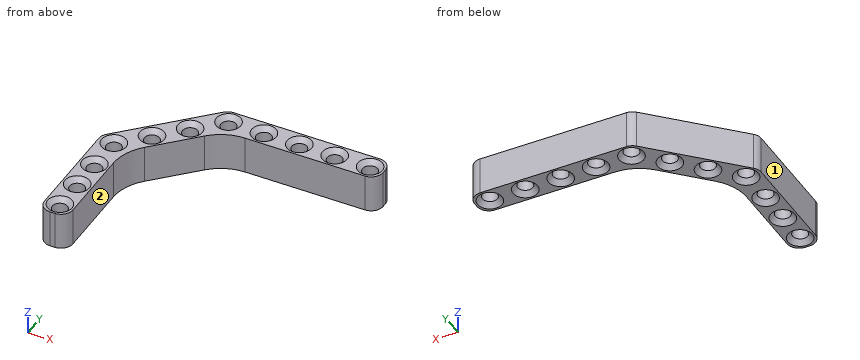
```python
from build123d import *

# Parameters (mm, degrees)
SKETCH1_R           = 1.6
BOSS_EXTRUDE1_DEPTH = 8
CHAMFER1_SIZE       = 1
SKETCH2_R           = 1.6
BOSS_EXTRUDE3_DEPTH = 8
FILLET1_R           = 10
CHAMFER2_SIZE       = 1
SKETCH3_R           = 1.6
BOSS_EXTRUDE4_DEPTH = 8
CHAMFER5_SIZE       = 1
FILLET2_R           = 10


with BuildPart() as part:
    # Sketch1 → Boss-Extrude1 (new body)
    with BuildSketch(Plane.XY):
        with BuildLine():
            Line((-0.5, 3), (30.5, 3))
            ThreePointArc((30.5, 3), (32.267766953, 2.267766953), (33, 0.5))
            Line((33, 0.5), (33, -0.5))
            ThreePointArc((33, -0.5), (32.267766953, -2.267766953), (30.5, -3))
            Line((30.5, -3), (-0.5, -3))
            ThreePointArc((-0.5, -3), (-2.267766953, -2.267766953), (-3, -0.5))
            Line((-3, -0.5), (-3, 0.5))
            ThreePointArc((-3, 0.5), (-2.267766953, 2.267766953), (-0.5, 3))
        make_face()
        Circle(SKETCH1_R, mode=Mode.SUBTRACT)
        with Locations((7.5, 0)):
            Circle(SKETCH1_R, mode=Mode.SUBTRACT)
        with Locations((15, 0)):
            Circle(SKETCH1_R, mode=Mode.SUBTRACT)
        with Locations((22.5, 0)):
            Circle(SKETCH1_R, mode=Mode.SUBTRACT)
        with Locations((30, 0)):
            Circle(SKETCH1_R, mode=Mode.SUBTRACT)
    extrude(amount=BOSS_EXTRUDE1_DEPTH)

    # Chamfer1
    chamfer1_edges = [part.edges().sort_by_distance(p)[0] for p in [
        (-1.6, 0, 0),
        (-1.6, 0, 8),
        (5.9, 0, 0),
        (5.9, 0, 8),
        (13.4, 0, 0),
        (13.4, 0, 8),
        (20.9, 0, 0),
        (20.9, 0, 8),
        (28.4, 0, 0),
        (28.4, 0, 8),
    ]]
    chamfer(chamfer1_edges, length=CHAMFER1_SIZE)

    # Sketch2 → Boss-Extrude3 (add)
    with BuildSketch(Plane.XY.offset(8)):
        with BuildLine():
            ThreePointArc((-3, 0.5), (-2.809698831, 1.456708581), (-2.267766953, 2.267766953))
            Line((-2.267766953, 2.267766953), (-18.529200529, -13.993666623))
            ThreePointArc((-18.529200529, -13.993666623), (-19.261433576, -15.761433576), (-18.529200529, -17.529200529))
            Line((-18.529200529, -17.529200529), (-17.822093748, -18.23630731))
            ThreePointArc((-17.822093748, -18.23630731), (-16.054326795, -18.968540357), (-14.286559842, -18.23630731))
            Line((-14.286559842, -18.23630731), (0.949747468, -3))
            Line((0.949747468, -3), (-0.5, -3))
            ThreePointArc((-0.5, -3), (-2.267766953, -2.267766953), (-3, -0.5))
            Line((-3, -0.5), (-3, 0.5))
        make_face()
        with Locations((-16.054326795, -15.761433576)):
            Circle(SKETCH2_R, mode=Mode.SUBTRACT)
        with Locations((-10.751025936, -10.458132717)):
            Circle(SKETCH2_R, mode=Mode.SUBTRACT)
        with Locations((-5.447725077, -5.154831858)):
            Circle(SKETCH2_R, mode=Mode.SUBTRACT)
    extrude(amount=-BOSS_EXTRUDE3_DEPTH)

    # Fillet1
    fillet1_edges = [part.edges().sort_by_distance(p)[0] for p in [
        (0.949747468, -3, 4),
    ]]
    fillet(fillet1_edges, radius=FILLET1_R)

    # Chamfer2
    chamfer2_edges = [part.edges().sort_by_distance(p)[0] for p in [
        (-17.654326795, -15.761433576, 8),
        (-12.351025936, -10.458132717, 8),
        (-7.047725077, -5.154831858, 8),
        (-7.047725077, -5.154831858, 0),
        (-12.351025936, -10.458132717, 0),
        (-17.654326795, -15.761433576, 0),
    ]]
    chamfer(chamfer2_edges, length=CHAMFER2_SIZE)

    # Sketch3 → Boss-Extrude4 (add)
    with BuildSketch(Plane.XY.offset(8)):
        with BuildLine():
            ThreePointArc((-18.529200529, -17.529200529), (-19.071132407, -16.718142157), (-19.261433576, -15.761433576))
            Line((-19.261433576, -15.761433576), (-19.261433576, -37.761433576))
            ThreePointArc((-19.261433576, -37.761433576), (-18.529200529, -39.529200529), (-16.761433576, -40.261433576))
            Line((-16.761433576, -40.261433576), (-15.761433576, -40.261433576))
            ThreePointArc((-15.761433576, -40.261433576), (-13.993666623, -39.529200529), (-13.261433576, -37.761433576))
            Line((-13.261433576, -37.761433576), (-13.261433576, -17.211181044))
            Line((-13.261433576, -17.211181044), (-14.286559842, -18.23630731))
            ThreePointArc((-14.286559842, -18.23630731), (-16.054326795, -18.968540357), (-17.822093748, -18.23630731))
            Line((-17.822093748, -18.23630731), (-18.529200529, -17.529200529))
        make_face()
        with Locations((-16.261433576, -30.261433576)):
            Circle(SKETCH3_R, mode=Mode.SUBTRACT)
        with Locations((-16.261433576, -37.261433576)):
            Circle(SKETCH3_R, mode=Mode.SUBTRACT)
        with Locations((-16.261433576, -23.261433576)):
            Circle(SKETCH3_R, mode=Mode.SUBTRACT)
    extrude(amount=-BOSS_EXTRUDE4_DEPTH)

    # Chamfer5
    chamfer5_edges = [part.edges().sort_by_distance(p)[0] for p in [
        (-17.861433576, -37.261433576, 8),
        (-17.861433576, -30.261433576, 8),
        (-17.861433576, -23.261433576, 8),
        (-17.861433576, -23.261433576, 0),
        (-17.861433576, -30.261433576, 0),
        (-17.861433576, -37.261433576, 0),
    ]]
    chamfer(chamfer5_edges, length=CHAMFER5_SIZE)

    # Fillet2
    fillet2_edges = [part.edges().sort_by_distance(p)[0] for p in [
        (-13.261433576, -17.211181044, 4),
    ]]
    fillet(fillet2_edges, radius=FILLET2_R)


solid = part.part
```
Can you work these out from the model? Positions are in its coordinate system, mm. Face numbers are marked on the shaded views. A direction names the side the tool comes from. Coordinates: 2 decimals unless noted, no trailing zeros. Write each loop counter-clockwise with the first axis right and the second up, starting at its lowest first coordinate (ties: lowest second). Pieces come first, ordered by that corner, then holes. Notation, with made-up numbers: (55.5, -17) - (76.5, -17) arc R16 cw to (76.5, -5) - close; hole circle Ø5 at (-27, -25.5). An arc over 180 degrees is marked (long way). Return JSON: item names as keys, results as strings.
Q1. Please list where these lines run through material, in increasing order: L1, parallel to Y at x = 22.5, z = 3.05; L2, parallel to X at y = -1, z = 4; L3, parallel to X at y = -29, z = 2.5. Write a range as from..to.
Computed values:
{"L1": "y = -3..-1.6, 1.6..3", "L2": "x = -5.54..-1.25, 1.25..6.25, 8.75..13.75, 16.25..21.25, 23.75..28.75, 31.25..32.95", "L3": "x = -19.26..-17.25, -15.28..-13.26"}
Q2. I'm going to push flat-ended pins straight in: pin 1 Ø1.5 at (y, z) = (-34, 5) entering from +X; pin 2 Ø5 at (x, y) = (-16.05, -15.76) entering from +Z; pin 3 Ø4 at (x, y) = (-10.75, -10.46) entering from +Z. Where does each tip first touch, or does it pass through?
Computed values:
{"pin 1": "stops at x = -13.26", "pin 2": "stops at z = 7.9", "pin 3": "stops at z = 7.4"}
Q3. On a 3-axis mill with a long thin cutter (end or side, diameter ignored), from which of +Z, -Z, +X, -X, +Y, -Y can I reach the whole of each face in a straight line? I mean the marked faces 1 and 2. Say none if no direction works.
Computed values:
{"face 1": "+Z, -Z, -X, +Y, -Y", "face 2": "+Z, -Z, +X, -Y"}
Q4. If we section it at A-A (x = 7.5): Please give me the cut outline in (y, z), then the cut area to 3 significant figures.
Computed values:
{"outline": "(-3, 0) - (-2.6, 0) - (-1.6, 1) - (-1.6, 7) - (-2.6, 8) - (-3, 8) - close; (1.6, 1) - (2.6, 0) - (3, 0) - (3, 8) - (2.6, 8) - (1.6, 7) - close", "area": "20.4 mm2"}
Q5. If we section it at B-B (z = 2.25): Count the separate pieces of the cut face and the enclosed holes in it, then the cut area to 3 significant figures.
Computed values:
{"separate pieces": "1", "enclosed holes": "11", "area": "391 mm2"}
